from build123d import *

# Parameters (mm, degrees)
SKETCH1_R           = 5.525
SKETCH1_R_2         = 1.75
BOSS_EXTRUDE1_DEPTH = 6.91


with BuildPart() as part:
    # Sketch1 → Boss-Extrude1 (new body)
    with BuildSketch(Plane.XY):
        with BuildLine():
            Line((27.759212348, 19.618292738), (53.215056471, 19.618292738))
            ThreePointArc((53.215056471, 19.618292738), (53.559180072, 19.658299948), (53.884947106, 19.776187475))
            ThreePointArc((53.884947106, 19.776187475), (66.467896523, 31.618292738), (70.431985807, 48.436499219))
            ThreePointArc((70.431985807, 48.436499219), (70.371195883, 48.77756551), (70.233781342, 49.095588895))
            Line((70.233781342, 49.095588895), (57.505859281, 71.14099658))
            ThreePointArc((57.505859281, 71.14099658), (57.299150221, 71.419012756), (57.03417311, 71.642191519))
            ThreePointArc((57.03417311, 71.642191519), (40.48713441, 76.618292738), (23.940095709, 71.642191519))
            ThreePointArc((23.940095709, 71.642191519), (23.675118599, 71.419012756), (23.468409538, 71.14099658))
            Line((23.468409538, 71.14099658), (10.732258497, 49.081335884))
            ThreePointArc((10.732258497, 49.081335884), (10.618509348, 48.835351928), (10.550877955, 48.572915326))
            ThreePointArc((10.550877955, 48.572915326), (11.255747963, 47.20128209), (12.797690777, 47.176146091))
            Line((12.797690777, 47.176146091), (13.260683436, 47.443455028))
            ThreePointArc((13.260683436, 47.443455028), (18.724785051, 45.979353412), (17.260683436, 40.515251797))
            Line((17.260683436, 40.515251797), (12.998198083, 38.054304731))
            ThreePointArc((12.998198083, 38.054304731), (12.337555741, 37.265255041), (12.340885644, 36.236159988))
            ThreePointArc((12.340885644, 36.236159988), (18.144128021, 26.598550843), (27.089321713, 19.776187475))
            ThreePointArc((27.089321713, 19.776187475), (27.415088747, 19.658299948), (27.759212348, 19.618292738))
        make_face()
        with Locations((33.270256045, 34.118292738)):
            Circle(SKETCH1_R, mode=Mode.SUBTRACT)
        with Locations((54.920891139, 46.618292738)):
            Circle(SKETCH1_R, mode=Mode.SUBTRACT)
        with Locations((33.270256045, 59.118292738)):
            Circle(SKETCH1_R, mode=Mode.SUBTRACT)
        with Locations((40.48713441, 46.618292738)):
            Circle(SKETCH1_R, mode=Mode.SUBTRACT)
        with Locations((18.836499315, 34.118292738)):
            Circle(SKETCH1_R_2, mode=Mode.SUBTRACT)
        with Locations((62.137769504, 34.118292738)):
            Circle(SKETCH1_R_2, mode=Mode.SUBTRACT)
        with Locations((40.48713441, 71.618292738)):
            Circle(SKETCH1_R_2, mode=Mode.SUBTRACT)
        with BuildLine():
            Line((24.689235101, 41.401001388), (24.168290568, 44.355424648))
            ThreePointArc((24.168290568, 44.355424648), (23.12568023, 45.085468265), (22.395636613, 44.042857928))
            Line((22.395636613, 44.042857928), (22.916581146, 41.088434669))
            ThreePointArc((22.916581146, 41.088434669), (23.959191483, 40.358391051), (24.689235101, 41.401001388))
        make_face(mode=Mode.SUBTRACT)
        with BuildLine():
            Line((20.040174245, 51.505531858), (17.742040916, 53.433894687))
            ThreePointArc((17.742040916, 53.433894687), (16.474092068, 53.322963537), (16.585023219, 52.055014689))
            Line((16.585023219, 52.055014689), (18.883156548, 50.12665186))
            ThreePointArc((18.883156548, 50.12665186), (20.151105395, 50.237583011), (20.040174245, 51.505531858))
        make_face(mode=Mode.SUBTRACT)
    extrude(amount=BOSS_EXTRUDE1_DEPTH)


solid = part.part
Geometry check sheet. Reference: the model listing, model coordinates, mm. A direction names the side the tool comes from. Coordinates: 2 decimals unless noted, no trailing zeros. Order: outer loops, then holes, each group sorted by start corner. A loop starts at its lowest first (then second) coordinate and runs counter-clockwise, first axis right, second up. Notation, with made-up numbers: (-4, -18) - (15, -18) arc R17 cw to (15, 0) - close; hole circle Ø9 at (-9.75, 83.5). An arc over 180 degrees is marked (long way). Answer in a Markdown table with one row per item. Add a question column.
1) Cross-section at B-B, the plane x = 28.5. Record the cut outline in (y, z).
2) Gauge pin test, flat ends, axial feed: P1, Ø4, axis at y = 37.5, z = 3, coming from the +X side; P2, Ø9, axis at x = 54.92, y = 46.62, coming from the -Z side; P3, Ø1, axis at x = 61.5, z = 3.5, coming from the +Y side; P4, Ø4, axis at y = 55, z = 1, coming from the +X side. Record the tip position at first contact, or that the pin passes through.
3) Cross-section at C-C, the plane z = 6. State how many separate pieces and enclosed holes the cut face has, then the cut area to 3 significant figures.
4) Release check for a two-part mould opening along X. For faces 1 (the flat face through (47, 49, 6.91)), 2 (the flat face through (63.96, 59.96, 3.41)), 3 (the cylindrical face through (60.19, 48.28, 3.41)) record: +X half, -X half, draft (parallel to the pull), parting line (faces both ways), or undercut.
5) Cross-section at D-D, the plane y = 23. Record the cut outline in (x, z).
6) Material ranges on line 1 along Y through (x, z) = (36.5, 4.25); line 2 along Y through (x, z) = (32, 3.75); line 3 along Y through (x, z) = (16.5, 2), recorded low to high. Write a range as [from, to].
7) Set-up check for faces 4 (the flat face through (15.159, 39.302, 3.407)), 5 (the cylindrical face through (40.733, 76.617, 3.407)), 6 (the flat face through (18.907, 52.456, 3.407)): record each of +Z, -Z, +X, -X, +Y, -Y from which the full face is reachable in a straight line by a thin tool's end or side.
8) Cross-section at A-A, the plane x = 14. Record the cut outline in (y, z), then the cut area to 3 significant figures.
Check result:
| question | item | result |
|---|---|---|
| 1 | outline | (19.62, 0) - (31.33, 0) - (31.33, 6.91) - (19.62, 6.91) - close; (36.91, 0) - (56.33, 0) - (56.33, 6.91) - (36.91, 6.91) - close; (61.91, 0) - (74.12, 0) - (74.12, 6.91) - (61.91, 6.91) - close |
| 2 | P1 | stops at x = 69.63 |
| 2 | P2 | passes through |
| 2 | P3 | stops at y = 65.09 |
| 2 | P4 | stops at x = 67.98 |
| 3 | separate pieces | 1 |
| 3 | enclosed holes | 9 |
| 3 | area | 2,170 mm² |
| 4 | face 1 | draft |
| 4 | face 2 | +X half |
| 4 | face 3 | undercut |
| 5 | outline | (21.99, 0) - (58.99, 0) - (58.99, 6.91) - (21.99, 6.91) - close |
| 6 | line 1 | y = [19.62, 29.64], [38.6, 42.79], [50.44, 54.64], [63.6, 76.35] |
| 6 | line 2 | y = [19.62, 28.74], [39.5, 53.74], [64.5, 75.39] |
| 6 | line 3 | y = [28.6, 40.08], [47.78, 52.14], [53.35, 59.07] |
| 7 | face 4 | +Z, -Z, -X |
| 7 | face 5 | +Z, -Z, +Y |
| 7 | face 6 | +Z, -Z |
| 8 | outline | (32.53, 0) - (38.63, 0) - (38.63, 6.91) - (32.53, 6.91) - close; (47.78, 0) - (54.74, 0) - (54.74, 6.91) - (47.78, 6.91) - close |
| 8 | area | 90.3 mm² |
